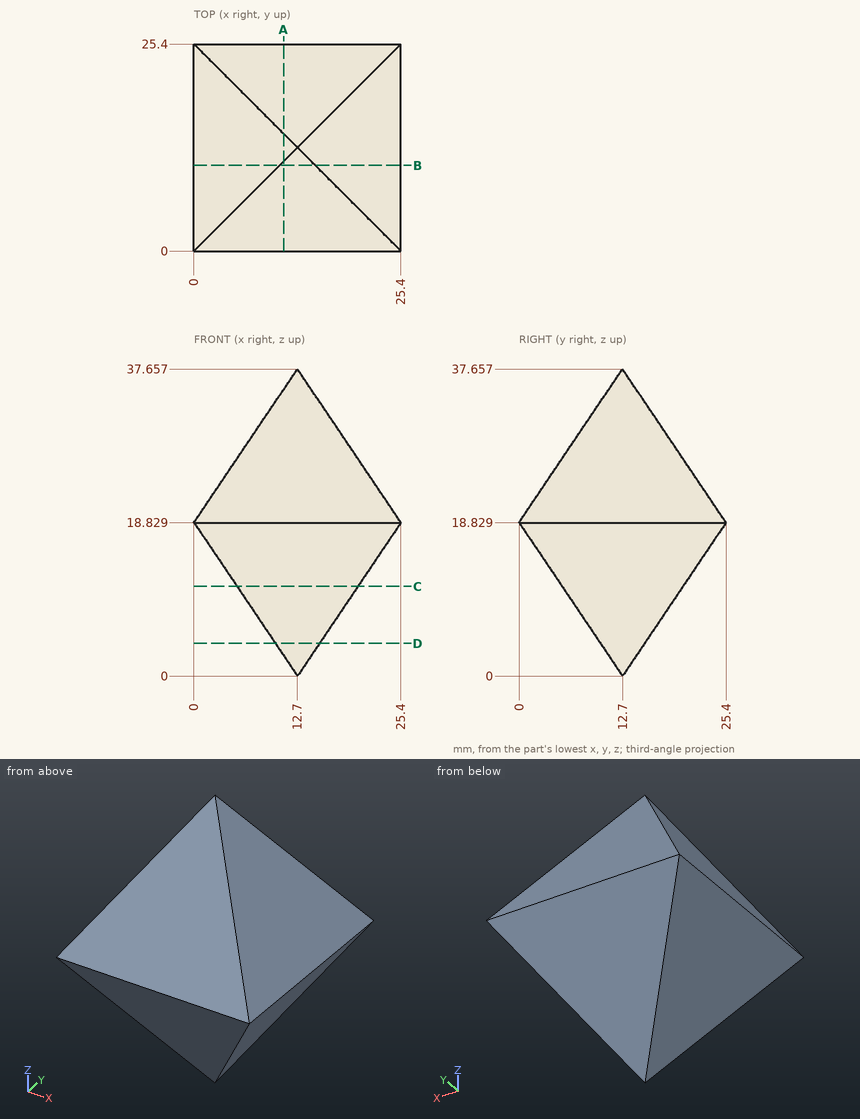
Job drawing, mm, ordinate dimensions from the low corner. One solid piece. Give positions to 0.01 mm unless a question says otherwise; leave off trailing zeros. Order: outer loops, then holes, each group sorted by start corner. A loop starts at its lowest first (then second) coordinate and runs counter-clockwise, first axis right, second up. Notation, with made-up numbers: (12, 49.5) - (30, 49.5) arc R32 cw to (30, 81.5) - close; hole circle Ø2 at (7.5, 57.25). An arc over 180 degrees is marked (long way). Answer in a Markdown table with one row per item.
1. Saw through at B-B, the plane y = 10.5. Give the cut face in (x, z) (1 decimal).
Data:
| item | result |
|---|---|
| outline | (0, 18.8) - (10.5, 3.3) - (14.9, 3.3) - (25.4, 18.8) - (14.9, 34.4) - (10.5, 34.4) - close |
2. Saw through at C-C, the plane z = 11. Give the cut face in (x, y), plus the area to 3 significant figures.
Data:
| item | result |
|---|---|
| outline | (5.28, 5.28) - (20.12, 5.28) - (20.12, 20.12) - (5.28, 20.12) - close |
| area | 220 mm² |
3. Saw through at D-D, the plane z = 4. Give the cut face in (x, y), plus the area to 3 significant figures.
Data:
| item | result |
|---|---|
| outline | (10, 10) - (15.4, 10) - (15.4, 15.4) - (10, 15.4) - close |
| area | 29.1 mm² |
4. Probe probe 1 along Z at (x, y) = (23.75, 24.25) (1 decimal); probe 2 along Z at (x, y) = (1.75, 15) (1 decimal); probe 3 along X at (y, z) = (10, 28.5) (1 decimal). List the from-to ranges inside material, lowest first. Write a range as [from, to].
Data:
| item | result |
|---|---|
| probe 1 | z = [17.1, 20.5] |
| probe 2 | z = [16.2, 21.4] |
| probe 3 | x = [6.5, 18.9] |
5. Flat gauge pins, fed straight in: pin 1 (1.5 mm diameter, centred on x = 18.5, y = 11, fed in from +Z); pin 2 (3 mm diameter, centred on y = 17.5, z = 26, fed in from +X) (1 decimal); pin 3 (3 mm diameter, centred on x = 5, y = 11, fed in from -Z). Where does each tip first touch, or does it go through?
Data:
| item | result |
|---|---|
| pin 1 | stops at z = 30.17 |
| pin 2 | stops at x = 21.6 |
| pin 3 | stops at z = 9.19 |
6. Saw through at A-A, the plane x = 11. Give the cut face in (y, z), plus the area to 3 significant figures.
Data:
| item | result |
|---|---|
| outline | (0, 18.83) - (11, 2.52) - (14.4, 2.52) - (25.4, 18.83) - (14.4, 35.14) - (11, 35.14) - close |
| area | 470 mm² |
